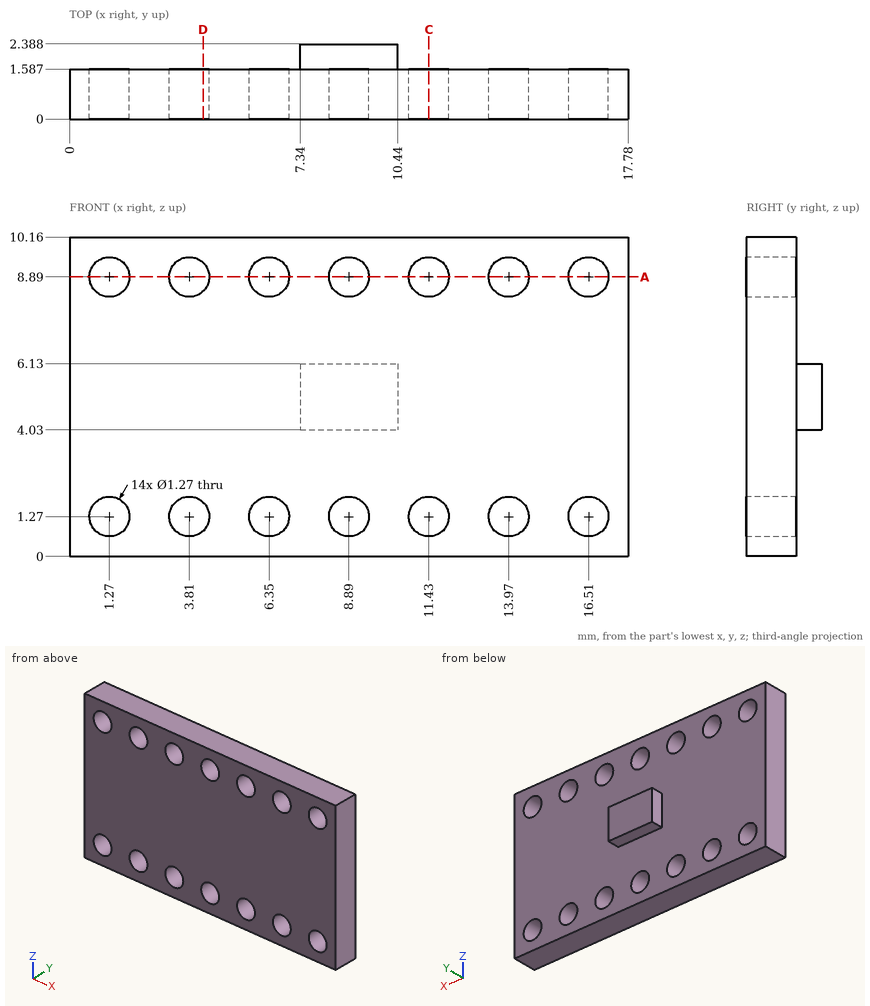
Here's the drawing with two shaded views (mm, measured from the low corner). I have some questions. Give positions to 0.01 mm unless a question says otherwise; leave off trailing zeros. Loops run counter-clockwise (first coordinate to the right, second up) from the corner with the lowest first, then second, coordinate; pieces in that order, holes last. Notation, with made-up numbers: M 79,-20.5 L 122,-20.5 A17 ccw 122,7.5 Z; hole C 85,5.25 d6. An arc over 180 degrees is marked long. One line per item, written item: value. Start each with the question number.
1) If we section it at D-D, the plane x = 4.25: Write out the boundary of the cut face in (y, z), and give its area (3 significant figures).
2) I'm going to push flat-ended pins straight in: pin 1 (0.8 mm diameter, centred on x = 8.89, z = 1.27, fed in from -Y); pin 2 (6 mm diameter, centred on x = 15, z = 6, fed in from +Y). Where does each tip first touch, or does it pass through?
3) If we section it at A-A, the plane z = 8.89: Give the number of separate pieces and of enclosed holes in the cut face.
4) If we section it at C-C, the plane x = 11.43: Write out the boundary of the cut face in (y, z) (1 decimal), and give its area (3 significant figures).
5) If I drill on line 1 (Z direction, x = 3.75, y = 1.3); line 2 (Z direction, x = 14.5, y = 0.9); line 3 (Y direction, x = 15.5, z = 9.5), over which ranges is the centre line in solid material (lowest first)? Write a range as [from, to].
Completed:
1. outline: M 0,0 L 1.59,0 L 1.59,0.81 L 0,0.81 Z; M 0,1.73 L 1.59,1.73 L 1.59,8.43 L 0,8.43 Z; M 0,9.35 L 1.59,9.35 L 1.59,10.16 L 0,10.16 Z
1. area: 13.2 mm^2
2. pin 1: passes through
2. pin 2: stops at y = 1.59
3. separate pieces: 8
3. enclosed holes: 0
4. outline: M 0,0 L 1.6,0 L 1.6,0.6 L 0,0.6 Z; M 0,1.9 L 1.6,1.9 L 1.6,8.3 L 0,8.3 Z; M 0,9.5 L 1.6,9.5 L 1.6,10.2 L 0,10.2 Z
4. area: 12.1 mm^2
5. line 1: z = [0, 0.64], [1.9, 8.26], [9.52, 10.16]
5. line 2: z = [0, 0.92], [1.62, 8.54], [9.24, 10.16]
5. line 3: y = [0, 1.59]
